Autodesk Inventor part; units mm, degrees
ref_plane "YZ Plane" through (0, 0, 0) normal (1, 0, 0) x (0, 1, 0)
ref_plane "XZ Plane" through (0, 0, 0) normal (0, 1, 0) x (-1, 0, 0)
ref_plane "XY Plane" through (0, 0, 0) normal (0, 0, 1) x (1, 0, 0)
sketch "Szkic1" plane through (0, 0, 0) normal (0, 1, 0) x (-1, 0, 0)
  line L0 (0, 0) -> (49, 0)
  line L1 (49, 0) -> (49, -45)
  line L2 (49, -45) -> (0, -45)
  line L3 (0, -45) -> (0, 0)
  line L4 (49, 0) -> (49, 3)
  line L5 (49, 3) -> (52, 3)
  line L6 (0, -45) -> (0, -48)
  line L7 (0, -48) -> (-3, -48)
  line L8 (-3, -48) -> (52, -48)
  line L9 (52, -48) -> (52, 3)
  line L10 (52, 3) -> (-3, 3)
  line L11 (-3, 3) -> (-3, -48)
  line L12 (0, -48) -> (-29.5685, -48)
  line L13 (-29.5685, -48) -> (-29.5685, 3)
  line L14 (-29.5685, 3) -> (0, 3)
  line L15 (0, 3) -> (0, -48)
  line L16 (-3, -45) -> (-29.5685, -45)
  line L17 (-3, 0) -> (-29.5685, 0)
  line L18 (-3, 0) -> (0, 0)
  line L19 (0, -45) -> (-3, -45)
  line L20 (-3, -45) -> (-3, -48)
  line L21 (0, -48) -> (0, -45)
  line L22 (0, -48) -> (-3, -48)
  dimension "d0" = 49
  dimension "d1" = 45
  dimension "d2" = 3
  dimension "d3" = 3
  dimension "d4" = 3
  dimension "d5" = 3
extrude "Wyciągnięcie proste1" add sketch "Szkic1" along normal blind 37.2 contours L0 L1 L2 L3 | L3 L19 L11 L18 | L11 L16 L13 L17
sketch "Szkic2" plane through (0, 0, 0) normal (0, -1, 0) x (1, 0, 0)
  line L0 (-49, 0) -> (0, 0)
  line L1 (-24.5, 0) -> (-24.5, -45)
  line L2 (0, -45) -> (-49, -45)
  line L3 (-49, -45) -> (-49, 0)
  line L4 (-49, -22.5) -> (0, -22.5)
  line L5 (0, 0) -> (0, -45)
  circle A0 centre (-24.5, -22.5) radius 2.85
  circle A1 centre (-24.5, -22.5) radius 3
  dimension "d8" = 5.7
  dimension "d27" = 6
extrude "Wyciągnięcie proste2" cut sketch "Szkic2" against normal through all contours A1 L4 A0 L1 | L1 A0 L4 A1 | L4 A0 L1 A1 | A0 L4 L1 | L1 L4 A0 | A1 L1 A0 L4 | L4 L1 A0 | L4 A0 L1
sketch "Szkic3" plane through (0, 0, 0) normal (0, -1, 0) x (1, 0, 0)
  circle A0 centre (-24.5, -22.5) radius 2.85
  line L0 (-24.5, -22.5) -> (-37.8, -22.5)
  line L1 (-24.5, -22.5) -> (9, -22.5)
  line L2 (-37.8, -22.5) -> (9, -22.5)
  line L3 (9, -22.5) -> (9, -32.4)
  line L4 (9, -32.4) -> (-37.8, -32.4)
  line L5 (-37.8, -32.4) -> (-37.8, -22.5)
  line L6 (9, -22.5) -> (-37.8, -22.5)
  line L7 (-37.8, -22.5) -> (-37.8, -13.6)
  line L8 (-37.8, -13.6) -> (9, -13.6)
  line L9 (9, -13.6) -> (9, -22.5)
  line L10 (9, -32.4) -> (-37.8, -32.4)
  line L11 (9, -32.4) -> (13, -32.4)
  line L12 (-37.8, -13.6) -> (-41.8, -13.6)
  line L13 (13, -32.4) -> (13, -32.9)
  line L14 (-41.8, -13.6) -> (-41.8, -13)
  line L15 (13, -32.4) -> (13, -33)
  line L16 (-41.8, -13) -> (-42.5873, -13)
  line L17 (13, -33) -> (13.5, -33)
  line L18 (13.5, -33) -> (-42.5873, -33)
  line L19 (-42.5873, -33) -> (-42.5873, -13)
  line L20 (-42.5873, -13) -> (13.5, -13)
  line L21 (13.5, -13) -> (13.5, -33)
  line L22 (13.5, -13) -> (-6.5, -13)
  line L23 (-6.5, -13) -> (-6.5, -32.4)
  line L24 (-6.5, -32.4) -> (13.5, -32.4)
  line L25 (13.5, -32.4) -> (13.5, -13)
  line L26 (-37.8, -22.5) -> (-6.5, -22.5)
  line L27 (-6.5, -22.5) -> (-6.5, -16.35)
  line L28 (-6.5, -16.35) -> (-37.8, -16.35)
  line L29 (-37.8, -16.35) -> (-37.8, -22.5)
  line L30 (-37.8, -22.5) -> (-6.5, -22.5)
  line L31 (-6.5, -22.5) -> (-6.5, -28.65)
  line L32 (-6.5, -28.65) -> (-37.8, -28.65)
  line L33 (-37.8, -28.65) -> (-37.8, -22.5)
  line L34 (-6.5, -16.35) -> (-5.5, -16.35)
  line L35 (-5.5, -16.35) -> (-5.5, -28.65)
  line L36 (-5.5, -28.65) -> (-6.5, -28.65)
  line L37 (-6.5, -28.65) -> (-6.5, -16.35)
  line L38 (-37.8, -22.5) -> (-26.4, -22.5)
  line L39 (-24.5, -22.5) -> (-26.9, -22.5)
  circle A1 centre (-26.9, -22.5) radius 2.4
  point P0 (0, 0)
  dimension "d21" = 4
  dimension "d22" = 4
  dimension "d23" = 0.5
  dimension "d24" = 0.6
  dimension "d25" = 0.6
  dimension "d26" = 0.5
  dimension "d28" = 20
  dimension "d29" = 6.15
  dimension "d30" = 6.15
  dimension "d31" = 1
  dimension "d32" = 11.4
  dimension "d33" = 2.4
  dimension "d34" = 4.8
extrude "Wyciągnięcie proste3" cut sketch "Szkic3" against normal blind 37 contours L1 L23 L32 L5 L0 A1 A0 | A0 A1 L0 L7 L28 L23 L1 | A0 L0 A1 | A1 L0 A0 | L23 L34 L35 L1 | L1 L35 L36 L23 | L24 L21 L17 L15 L13 picked at (-27.9524, -22.0946) picked at (-27.9524, -22.9054)
sketch "Szkic4" plane through (0, 0, 0) normal (0, -1, 0) x (1, 0, 0)
  line L0 (-49, -45) -> (-49, 0)
  line L1 (-37.8, -28.65) -> (-37.8, -16.35)
  line L2 (-49, -22.5) -> (-37.8, -22.5)
  line L3 (-37.8, -22.5) -> (-37.8, -17.5)
  line L4 (-37.8, -17.5) -> (-49, -17.5)
  line L5 (-49, -17.5) -> (-49, -22.5)
  line L6 (-49, -22.5) -> (-37.8, -22.5)
  line L7 (-37.8, -22.5) -> (-37.8, -27.5)
  line L8 (-37.8, -27.5) -> (-49, -27.5)
  line L9 (-49, -27.5) -> (-49, -22.5)
  point P0 (0, 0)
  point P1 (-37.8, -32.4)
  point P2 (-37.8, -13.6)
  dimension "d17" = 5
  dimension "d18" = 5
extrude "Wyciągnięcie proste4" cut sketch "Szkic4" against normal blind 10
sketch "Szkic5" plane through (0, 37, 0) normal (0, -1, 0) x (1, 0, 0)
  line L0 (-37.8, -28.65) -> (-37.8, -16.35)
  line L1 (-37.8, -22.5) -> (-26.3, -22.5)
  line L2 (-26.3, -22.5) -> (-28.7, -22.5)
  circle A0 centre (-28.7, -22.5) radius 2.4
  point P0 (0, 0)
  dimension "d35" = 11.5
  dimension "d36" = 2.4
  dimension "d37" = 4.8
extrude "Wyciągnięcie proste5" cut sketch "Szkic5" against normal blind 37
sketch "Szkic6" plane through (0, 37, 0) normal (0, -1, 0) x (1, 0, 0)
  arc A0 (-26.9857, -20.8203) -> (-26.9857, -24.1797) centre (-28.7, -22.5) ccw
  circle A1 centre (-28.7, -22.5) radius 2.4
  arc A2 (-26.9857, -24.1797) -> (-26.9857, -20.8203) centre (-24.5, -22.5) ccw
  circle A3 centre (-24.5, -22.5) radius 3
  point P0 (0, 0)
extrude "Wyciągnięcie proste6" add sketch "Szkic6" against normal blind 0.2 contours A2 A1
sketch "Szkic7" plane through (0, 0, 0) normal (0, -1, 0) x (1, 0, 0)
  line L0 (-49, 0) -> (29.5685, 0)
  line L1 (-49, 0) -> (0, 0)
  line L2 (29.5685, 0) -> (29.5685, -45)
  line L3 (0, 0) -> (29.5685, 0)
  line L4 (29.5685, 0) -> (29.5685, -45)
  line L5 (29.5685, -45) -> (0, -45)
  line L6 (0, -45) -> (0, 0)
  dimension "d42" = 49
extrude "Wyciągnięcie proste7" cut sketch "Szkic7" against normal through all
sketch "Szkic8" plane through (0, 0, 0) normal (0, -1, 0) x (1, 0, 0)
  line L0 (-49, -45) -> (-49, 0)
  line L1 (0, 0) -> (0, -45)
  line L2 (-49, 0) -> (0, 0)
  line L3 (0, 0) -> (0, -45)
  line L4 (0, -45) -> (-49, -45)
  line L5 (-49, -45) -> (-49, 0)
sketch "Szkic9" plane through (-49, 0, 0) normal (0, 0, 1) x (1, 0, 0)
  line L0 (0, 37.2) -> (0, 9.2)
  line L1 (0, 0) -> (0, 37.2)
  point P0 (49, 0)
  dimension "d45" = 28
extrude "Wyciągnięcie proste8" cut sketch "Szkic8" against normal blind 9.2
sketch "Szkic10" plane through (0, 10, 0) normal (0, -1, 0) x (1, 0, 0)
  line L0 (-49, -45) -> (-49, -27.5)
  line L1 (-37.8, -28.65) -> (-37.8, -16.35)
  line L2 (-49, -27.5) -> (-37.8, -27.5)
  line L3 (-37.8, -27.5) -> (-37.8, -17.4794)
  line L4 (-37.8, -17.4794) -> (-49, -17.4794)
  line L5 (-49, -17.4794) -> (-49, -27.5)
  point P0 (0, 0)
extrude "Wyciągnięcie proste9" cut sketch "Szkic10" against normal blind 5.55
sketch "Szkic11" plane through (0, 37.2, 0) normal (0, 1, 0) x (1, 0, 0)
  circle A0 centre (-28.7, 22.5) radius 2.4
  circle A1 centre (-28.7, 22.5) radius 2.4
  line L0 (-49, 45) -> (-49, 27.5)
  line L1 (0, 0) -> (-49, 0)
  line L2 (-49, 0) -> (-49, 45)
  line L3 (-49, 45) -> (0, 45)
  line L4 (0, 45) -> (0, 0)
extrude "Wyciągnięcie proste10" add sketch "Szkic11" along normal blind 1
sketch "Szkic12" plane through (0, 9.2, 0) normal (0, -1, 0) x (1, 0, 0)
  line L0 (0, -45) -> (-49, -45)
  line L1 (-49, 0) -> (0, 0)
  line L2 (0, 0) -> (0, -45)
  line L3 (0, -45) -> (-49, -45)
  line L4 (-49, -45) -> (-49, 0)
extrude "Wyciągnięcie proste11" cut sketch "Szkic12" against normal blind 1.5
sketch "Szkic13" plane through (0, 38.2, 0) normal (0, 1, 0) x (1, 0, 0)
  line L0 (-49, 45) -> (-49, 0)
  line L1 (-49, 22.5) -> (-26, 22.5)
  line L2 (-26, 22.5) -> (-28.4, 22.5)
  circle A0 centre (-28.4, 22.5) radius 2.5
  circle A1 centre (-26, 22.5) radius 2.5
  circle A2 centre (-27.2, 22.5) radius 2.5
  line L3 (-23.5, 20) -> (-31.1111, 20)
  line L4 (-31.1111, 20) -> (-31.1111, 25)
  line L5 (-31.1111, 25) -> (-23.5, 25)
  line L6 (-23.5, 25) -> (-23.5, 20)
  point P0 (0, 0)
  dimension "d54" = 23
  dimension "d55" = 2.4
  dimension "d56" = 5
  dimension "d57" = 5
  dimension "d58" = 5
extrude "Wyciągnięcie proste12" cut sketch "Szkic13" against normal blind 1.5
sketch "Szkic14" plane through (0, 38.2, 0) normal (0, 1, 0) x (1, 0, 0)
  line L0 (-54.5366, 52.5987) -> (6.0904, 52.5987)
  line L1 (6.0904, 52.5987) -> (6.0904, -5.7213)
  line L2 (6.0904, -5.7213) -> (-54.5366, -5.7213)
  line L3 (-54.5366, -5.7213) -> (-54.5366, 52.5987)
  point P0 (0, 0)
extrude "Wyciągnięcie proste13" cut sketch "Szkic14" against normal blind 0.3
Can you work these out from the model? Positions are in its coordinate system, mm. A direction names the side the tool comes from. Round coordinates to 2 decimals unless told otherwise and drop trailing zeros. Loops run counter-clockwise (first coordinate to the right, second up) from the corner with the lowest first, then second, coordinate; pieces in that order, holes last. Notation, with made-up numbers: (32.5, 38.25) - (40.5, 38.25) arc R26 cw to (40.5, 55.25) - close; hole circle Ø2 at (89, -38). An arc over 180 degrees is marked (long way). Answer in a Markdown table with one row per item. Add a question column.
Q1. I want a section at D-D on y = 14.5. List the corners of the cut face in (x, z) for me.
Q2. Which directions (+Z, -Z, +X, -X, +Y, -Y) give clear straight access to the entire face, cutting with the end or side of a thin tool? Please do faces 1 (the flat face through (-25, 37.9, -28)), 2 (the flat face through (-22, 37, -22)), 3 (the flat face through (-43, 13, -27.5)).
Q3. I need wall thicknesses on L1, parallel to Z at x = -8.5, y = 22.75; L2, parallel to Z at x = -46, y = 15.25; L3, parallel to X at y = 34, z = -18. Which ranges of each line are inside material? Lowest first, please.
Q4. We'd pull the mould along X, two halves only. Please class faces 4 (the flat face through (-43, 13, -17.479)), 5 (the flat face through (-49, 24, -23)), 6 (the flat face through (-5.5, 24, -22)): pulls with the +X half, pulls with the -X half, needs draft (parallel to the pull), parting line crosses it, or undercut.
Q5. I want a section at B-B on x = -30. List the corners of the cut face in (y, z) for me, and give its area (3 significant figures).
Q6. I want a section at C-C on x = -45. List the corners of the cut face in (y, z) for me, and give its area (3 significant figures).
Q7. I want a section at A-A on y = 31.5. List the corners of the cut face in (x, z) for me.
A:
| question | item | result |
|---|---|---|
| 1 | outline | (-49, -45) - (0, -45) - (0, 0) - (-49, 0) - (-49, -17.48) - (-37.8, -17.48) - (-37.8, -16.35) - (-5.5, -16.35) - (-5.5, -28.65) - (-37.8, -28.65) - (-37.8, -27.5) - (-49, -27.5) - close |
| 2 | face 1 | +Z, -Z, +X, -X, +Y |
| 2 | face 2 | -Y |
| 2 | face 3 | -X, -Y |
| 3 | L1 | -45 to -28.65, -16.35 to 0 |
| 3 | L2 | -45 to -27.5, -17.48 to 0 |
| 3 | L3 | -49 to -37.8, -5.5 to 0 |
| 4 | face 4 | needs draft |
| 4 | face 5 | pulls with the -X half |
| 4 | face 6 | undercut |
| 5 | outline | (10.7, -45) - (37.9, -45) - (37.9, -25) - (37, -25) - (37, -28.65) - (10.7, -28.65) - close; (10.7, -16.35) - (37, -16.35) - (37, -20) - (37.9, -20) - (37.9, 0) - (10.7, 0) - close |
| 5 | area | 896 mm^2 |
| 6 | outline | (10.7, -45) - (37.9, -45) - (37.9, 0) - (10.7, 0) - (10.7, -17.48) - (15.55, -17.48) - (15.55, -27.5) - (10.7, -27.5) - close |
| 6 | area | 1,180 mm^2 |
| 7 | outline | (-49, -45) - (0, -45) - (0, 0) - (-49, 0) - close; hole (-37.8, -28.65) - (-5.5, -28.65) - (-5.5, -16.35) - (-37.8, -16.35) - close |
